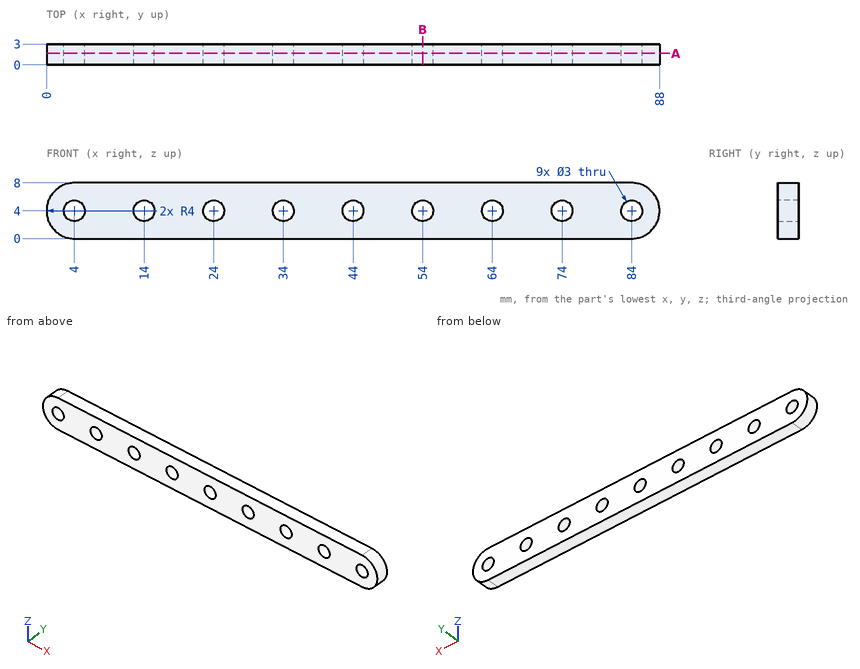
Input: dimensioned drawing with shaded views. Units: mm. Origin: part minimum x, y, z. Give positions to 0.01 mm unless a question says otherwise; leave off trailing zeros. Order: outer loops, then holes, each group sorted by start corner. A loop starts at its lowest first (then second) coordinate and runs counter-clockwise, first axis right, second up.
(1) Section query B-B (x = 54). Return the cut outline in (y, z), plus the area to 3 significant figures.
(2) Material intervals for line 1 along Z through (x, y) = (64, 2.35); line 2 along Z through (x, y) = (23, 1.75); line 3 along X through (y, z) = (1.2, 1.75), sorted ascending.
(3) Contact query for flat-ended pins moving along their axis: P1, Ø1.8, axis at x = 4, z = 4, coming from the -Y side; P2, Ø4, axis at x = 74, z = 4, coming from the +Y side; P3, Ø1.5, axis at y = 2.5, z = 5, coming from the +X side. Output: stop coordinate, or through.
(4) Section query A-A (y = 1.65). State how many separate pieces and enclosed holes the cut face has, plus the area to 3 significant figures.
Outcome:
1. outline: (0, 0) - (3, 0) - (3, 2.5) - (0, 2.5) - close; (0, 5.5) - (3, 5.5) - (3, 8) - (0, 8) - close
1. area: 15.0 mm2
2. line 1: z = 0 to 2.5, 5.5 to 8
2. line 2: z = 0 to 2.88, 5.12 to 8
2. line 3: x = 0.69 to 87.31
3. P1: passes through
3. P2: stops at y = 3
3. P3: stops at x = 87.99
4. separate pieces: 1
4. enclosed holes: 9
4. area: 627 mm2
